```python
from build123d import *

# Parameters (mm, degrees)
SZKIC2_R                   = 1
WYTNIJ_WYCI_GNI_CIE1_DEPTH = 2.9


with BuildPart() as part:
    # Szkic1 → Obrót1 (revolve)
    with BuildSketch(Plane.XY, mode=Mode.PRIVATE) as obr_t1_sk:
        Polygon((0, 0), (0, 2), (11.2, 2), (11.2, 5), (12.3, 5), (12.3, 13), (69.3, 13), (69.3, 5), (72.55, 5), (72.55, 1.5), (80.3, 1.5), (80.3, 0), align=None)
    revolve(obr_t1_sk.sketch.rotate(Axis((0, 0, 0), (-1, 0, 0)), 90), axis=Axis((0, 0, 0), (-1, 0, 0)))

    # Szkic2 → Wytnij-wyciągnięcie1 (cut)
    with BuildSketch(Plane(origin=(69.3, 0, 0), x_dir=(0, 0, -1), z_dir=(1, 0, 0))):
        with Locations((0, 8.5)):
            Circle(SZKIC2_R)
        with Locations((7.361215932, -4.25)):
            Circle(SZKIC2_R)
        with Locations((-7.361215932, -4.25)):
            Circle(SZKIC2_R)
    extrude(amount=-WYTNIJ_WYCI_GNI_CIE1_DEPTH, mode=Mode.SUBTRACT)


solid = part.part
```
Read the model definition and answer for the solid it produces. Units are mm, in the model's axes. A direction names the side the tool comes from. Give positions to 0.01 mm unless a question says otherwise; leave off trailing zeros. Order: outer loops, then holes, each group sorted by start corner. A loop starts at its lowest first (then second) coordinate and runs counter-clockwise, first axis right, second up.
(1) Find section B-B (y = 0). Give the vertices of the cut face in (x, z), plus the area to 3 significant figures.
(2) Given pin 1 (4 mm diameter, centred on x = 60.5, z = -8, fed in from +Y); pin 2 (5 mm diameter, centred on y = -1.5, z = -1.5, fed in from -X); pin 3 (1.5 mm diameter, centred on x = 57, z = 8.5, fed in from +Y); pin 4 (0.6 mm diameter, centred on y = -4.5, z = -7, fed in from +X), each flat-ended and moving along its own axis, determine where each tip first touches the part or whether it passes through.
(3) Straight lines are drawn through the part: L1, parallel to Y at x = 67.7, z = 0; L2, parallel to X at y = -1.75, z = -1.75; L3, parallel to X at y = 6.25, z = 8.5. For each, find the intervals that lie inside material, in ascending order.
(4) For a pull along Z with two mould halves and no side action, classify faces 4 (the cylindrical face through (67.87, -3.574, 8.098)), 5 (the flat face through (0, 0, 0)), 6 (the cylindrical face through (6, 2, 0)) as released by +Z, released by -Z, zero draft, split by the parting line, or undercut.
(5) For faces 1 (the cylindrical face through (67.9, -3.9, -8.3)), 2 (the flat face through (11.2, -0.1, 2.2)), 3 (the cylindrical face through (41.199, 7.91, 10.316)), determine the directions among +Z, -Z, +X, -X, +Y, -Y from which every point of the face is accessible in a straight line to the end or side of a thin tool.
(6) Find section A-A (z = 0). Give the vertices of the cut face in (x, y).
(7) Find section D-D (y = 3.5). Give the vertices of the cut face in (x, z), plus the area to 3 significant figures.
(8) Find section C-C (x = 31.5). Give the vertices of the cut face in (y, z).
Result sheet:
1. outline: (0, -2) - (11.2, -2) - (11.2, -5) - (12.3, -5) - (12.3, -13) - (69.3, -13) - (69.3, -5) - (72.55, -5) - (72.55, -1.5) - (80.3, -1.5) - (80.3, 1.5) - (72.55, 1.5) - (72.55, 5) - (69.3, 5) - (69.3, 13) - (12.3, 13) - (12.3, 5) - (11.2, 5) - (11.2, 2) - (0, 2) - close
1. area: 1,590 mm2
2. pin 1: stops at y = 11.53
2. pin 2: stops at x = 0
2. pin 3: stops at y = 10.44
2. pin 4: stops at x = 66.4
3. L1: y = -13 to 7.5, 9.5 to 13
3. L2: x = 11.2 to 72.55
3. L3: x = 12.3 to 69.3
4. face 4: undercut
4. face 5: zero draft
4. face 6: split by the parting line
5. face 1: +X
5. face 2: -X
5. face 3: +X, -X
6. outline: (0, -2) - (11.2, -2) - (11.2, -5) - (12.3, -5) - (12.3, -13) - (69.3, -13) - (69.3, -5) - (72.55, -5) - (72.55, -1.5) - (80.3, -1.5) - (80.3, 1.5) - (72.55, 1.5) - (72.55, 5) - (69.3, 5) - (69.3, 7.5) - (66.4, 7.5) - (66.4, 9.5) - (69.3, 9.5) - (69.3, 13) - (12.3, 13) - (12.3, 5) - (11.2, 5) - (11.2, 2) - (0, 2) - close
7. outline: (11.2, -3.57) - (12.3, -3.57) - (12.3, -12.52) - (69.3, -12.52) - (69.3, -3.57) - (72.55, -3.57) - (72.55, 3.57) - (69.3, 3.57) - (69.3, 12.52) - (12.3, 12.52) - (12.3, 3.57) - (11.2, 3.57) - close
7. area: 1,460 mm2
8. outline: circle Ø26 at (0, 0)
